Can you work these out from the model? Positions are in its coordinate system, mm. A direction names the side the tool comes from. Round coordinates to 2 decimals unless told otherwise and drop trailing zeros. Write each loop counter-clockwise with the first axis right and the second up, starting at its lowest first coordinate (ties: lowest second). Pieces come first, ordered by that corner, then holes. Notation, with made-up numbers: (-4.75, -1.75) - (39.25, -1.75) arc R27 ccw to (39.25, 32.25) - close; hole circle Ø10 at (11.5, 49.25). An arc over 180 degrees is marked (long way). One line per item, written item: value. Start each with the question number.
(1) I want a section at C-C on y = -9. List the corners of the cut face in (x, z) for me, plus the area to 3 significant figures.
(2) If I drill on L1, parallel to Z at x = 36.1, y = 0.3; L2, parallel to Z at x = -36.1, y = 0.85; L3, parallel to Y at x = -31, z = 5.75, over which ranges is the centre line in solid material (lowest first)? Write a range as from..to.
(3) I want a section at A-A on x = 12. List the corners of the cut face in (y, z) for me, plus the area to 3 significant figures.
(4) I'm going to push flat-ended pins straight in: pin 1 Ø3 at (x, z) = (6, 1) entering from -Y; pin 2 Ø0.8 at (y, z) = (-0.5, -4.5) entering from -X; pin 3 Ø0.9 at (y, z) = (-2, -4.5) entering from +X; pin 4 Ø3.5 at (x, y) = (0.5, -1) entering from +Z. Where does each tip first touch, or does it pass through?
(5) I want a section at B-B on z = 0. List the corners of the cut face in (x, y) for me, plus the area to 3 significant figures.
(6) I want a section at D-D on x = -36.1. List the corners of the cut face in (y, z) for me, plus the area to 3 significant figures.
(7) On a 3-axis mill with a long thin cutter (end or side, diameter ignored), from which of +Z, -Z, +X, -X, +Y, -Y can I reach the whole of each face in a straight line? I mean faces 4 (the face through (0, -1, -2.45)), 5 (the face through (-4, -1, 4)), 6 (the face through (-5, -1, -5)), 7 (the face through (-1, 1, 7.75)), 8 (the face through (-23, -1, 5)). Say none if no direction works.
(8) Thinking about a two-plate mould opening in X: for faces 1 (the face through (21, -1, -5)), 2 (the face through (38, 1, 0)), 3 (the face through (-1, 1, -7.75)), which applies, +X half, -X half, draft (parallel to the pull), parting line (faces both ways), or undercut?
from build123d import *

# Parameters (mm, degrees)
F0_W     = 76
F0_H     = 15.5
F0_R     = 1.1
F1_DEPTH = 1.2
F2_W     = 3.7
F2_H     = 4.3
F2_W_2   = 10
F2_H_2   = 4
F2_W_3   = 4.3
F2_H_3   = 3.7
F4_DEPTH = 1
F3_R     = 5
F5_DEPTH = 15
F6_W     = 10
F6_H     = 5.8
F7_DEPTH = 3


with BuildPart() as f1:
    # F0 (on Front) → F1 (new body)
    with BuildSketch(Plane.XZ):
        Rectangle(F0_W, F0_H)
        with Locations((36.1, -5.85)):
            Circle(F0_R, mode=Mode.SUBTRACT)
        with Locations((-36.1, 5.85)):
            Circle(F0_R, mode=Mode.SUBTRACT)
    extrude(amount=-F1_DEPTH)

    # F2 (on Front) → F4 (join)
    with BuildSketch(Plane.XZ):
        with Locations((11, -5.2)):
            Rectangle(F2_W, F2_H)
        with Locations((-23, 5.2)):
            Rectangle(F2_W, F2_H)
        with Locations((21, -5.2)):
            Rectangle(F2_W, F2_H)
        with Locations((-4, 3.75)):
            Rectangle(F2_W_2, F2_H_2)
        with Locations((-10.85, -4.4)):
            Rectangle(F2_W_3, F2_H_3)
    extrude(amount=F4_DEPTH)

    # F3 (on Front) → F5 (join)
    with BuildSketch(Plane.XZ):
        with Locations((32, 0)):
            Circle(F3_R)
        with Locations((-32, 0)):
            Circle(F3_R)
    extrude(amount=F5_DEPTH)

    # F6 (on Front) → F7 (join)
    with BuildSketch(Plane.XZ):
        with Locations((0, -5.35)):
            Rectangle(F6_W, F6_H)
    extrude(amount=F7_DEPTH)


solid = f1.part
Established:
1. outline: circle Ø10 at (-32, 0); circle Ø10 at (32, 0)
1. area: 157 mm2
2. L1: -7.75..-6.95, -4.75..7.75
2. L2: -7.75..4.75, 6.95..7.75
2. L3: 0..1.2
3. outline: (-1, -7.35) - (0, -7.35) - (0, -7.75) - (1.2, -7.75) - (1.2, 7.75) - (0, 7.75) - (0, -3.05) - (-1, -3.05) - close
3. area: 22.9 mm2
4. pin 1: y = 0
4. pin 2: x = -34.86
4. pin 3: x = 34.93
4. pin 4: z = 7.75
5. outline: (-38, 0) - (-37, 0) - (-37, -15) - (-27, -15) - (-27, 0) - (27, 0) - (27, -15) - (37, -15) - (37, 0) - (38, 0) - (38, 1.2) - (-38, 1.2) - close
5. area: 391 mm2
6. outline: (-15, -2.86) - (0, -2.86) - (0, -7.75) - (1.2, -7.75) - (1.2, 4.75) - (0, 4.75) - (0, 2.86) - (-15, 2.86) - close; (0, 6.95) - (1.2, 6.95) - (1.2, 7.75) - (0, 7.75) - close
6. area: 102 mm2
7. face 4: -Y
7. face 5: +Z, -Y
7. face 6: -Z, -Y
7. face 7: +Z, +X, -X, +Y, -Y
7. face 8: +Z, -Z, -Y
8. face 1: undercut
8. face 2: +X half
8. face 3: draft
